Part model, mm, in its own coordinate system. A direction names the side the tool comes from. Coordinates: 2 decimals unless noted, no trailing zeros. Write each loop counter-clockwise with the first axis right and the second up, starting at its lowest first coordinate (ties: lowest second). Pieces come first, ordered by that corner, then holes. Notation, with made-up numbers: (-6, 4.5) - (-2, 4.5) arc R33 cw to (-2, 38.5) - close; hole circle Ø3 at (-22, 22.25). An arc over 180 degrees is marked (long way). Write each question's results on one line, items separated by ' | '.
from build123d import *

# Parameters (mm, degrees)
F0_W     = 10
F0_H     = 5
F1_DEPTH = 1


with BuildPart() as f1:
    # F0 (on Front) → F1 (new body)
    with BuildSketch(Plane.XZ):
        Polygon((-0.377013, 15.377013), (-0.377013, 15), (0, 15), (0.377013, 15), (0.754026, 15.377013), (0.754026, 20), (-0.754026, 20), (-0.754026, 15.377013), align=None)
        with Locations((0, 2.5)):
            Rectangle(F0_W, F0_H)
        Polygon((-5, 25), (-0.754026, 20), (0.754026, 20), (5, 25), (5, 30), (-5, 30), align=None)
        Polygon((-0.754026, 10), (-5, 5), (5, 5), (0.754026, 10), align=None)
        Polygon((-0.754026, 14.622987), (-0.754026, 10), (0.754026, 10), (0.754026, 14.622987), (0.377013, 15), (0, 15), (-0.377013, 15), align=None)
        Polygon((-0.754026, 15.377013), (-0.377013, 15), (-0.377013, 15.377013), align=None)
    extrude(amount=F1_DEPTH)


solid = f1.part
(1) Saw through at A-A on x = -3. Write the cut outline in (y, z), then the cut area to 3 significant figures.
Return value:
outline: (-1, 0) - (0, 0) - (0, 7.36) - (-1, 7.36) - close; (-1, 22.64) - (0, 22.64) - (0, 30) - (-1, 30) - close | area: 14.7 mm^2
(2) Saw through at D-D on z = 12. Write the cut outline in (x, y).
Return value:
outline: (-0.75, -1) - (0.75, -1) - (0.75, 0) - (-0.75, 0) - close
(3) Two-plate mould, pull along Z, no slides. Class faces 1 (the flat face through (-0.1, -0.5, 0)), 2 (the flat face through (5, -0.5, 2.5)), 3 (the flat face through (-0.754, -0.5, 17.7)): released by +Z, released by -Z, zero draft, split by the parting line, or undercut.
Return value:
face 1: released by -Z | face 2: zero draft | face 3: undercut
(4) Saw through at C-C on x = 4. Write the cut outline in (y, z).
Return value:
outline: (-1, 0) - (0, 0) - (0, 6.18) - (-1, 6.18) - close; (-1, 23.82) - (0, 23.82) - (0, 30) - (-1, 30) - close
(5) 3-axis set-ups, long thin cutter, end or side, ignore diameter. For faces 4 (the flat face through (0.754, -0.5, 17.7)), 5 (the flat face through (-0.754, -0.5, 12.3)), 6 (the flat face through (-5, -0.5, 2.5)): which of +Z, -Z, +X, -X, +Y, -Y reach the whole face in a straight line?
Return value:
face 4: +X, +Y, -Y | face 5: -X, +Y, -Y | face 6: +Z, -Z, -X, +Y, -Y
(6) Saw through at B-B on y = -0.2. Write the cut outline in (x, z).
Return value:
outline: (-5, 0) - (5, 0) - (5, 5) - (0.75, 10) - (0.75, 14.62) - (0.38, 15) - (0.75, 15.38) - (0.75, 20) - (5, 25) - (5, 30) - (-5, 30) - (-5, 25) - (-0.75, 20) - (-0.75, 15.38) - (-0.38, 15) - (-0.75, 14.62) - (-0.75, 10) - (-5, 5) - close
(7) Wall check: line 1 (Z direction, x = 1.25, y = -0.45); line 2 (Z direction, x = -1, y = -0.65); line 3 (X direction, y = -0.5, z = 10.5). Give the ranges that are in metal, low to high. Write a range as from..to.
Return value:
line 1: z = 0..9.42, 20.58..30 | line 2: z = 0..9.71, 20.29..30 | line 3: x = -0.75..0.75
